```python
from build123d import *

# Parameters (mm, degrees)
SKETCH1_W           = 55
SKETCH1_H           = 25
BOSS_EXTRUDE1_DEPTH = 6
FILLET1_R           = 5


with BuildPart() as part:
    # Sketch1 → Boss-Extrude1 (new body)
    with BuildSketch(Plane.XY):
        Rectangle(SKETCH1_W, SKETCH1_H)
    extrude(amount=BOSS_EXTRUDE1_DEPTH)

    # Fillet1
    fillet1_edges = [part.edges().sort_by_distance(p)[0] for p in [
        (0, -12.5, 6),
    ]]
    fillet(fillet1_edges, radius=FILLET1_R)


solid = part.part
```
Model file for the job. Use its own axes, mm. Coordinates: 2 decimals unless noted, no trailing zeros. Write each loop counter-clockwise with the first axis right and the second up, starting at its lowest first coordinate (ties: lowest second). Pieces come first, ordered by that corner, then holes. Notation, with made-up numbers: (-11, -36) - (-2, -36) arc R17 cw to (-2, -24) - close; hole circle Ø3 at (27, 30). An arc over 180 degrees is marked (long way). One line per item, written item: value. Start each with the question number.
1. Slice it at A-A (x = -13). Write the cut outline in (y, z).
2. Flat gauge pin, fed straight in: pin 1 (1 mm diameter, centred on x = -13.5, z = 2.5, fed in from -Y). Where does the tip first touch, or does it go through?
3. Slice it at B-B (z = 5). Write the cut outline in (x, y), plus the area to 4 significant figures.
4. Probe line 1 (Y direction, x = 3.5, z = 3); line 2 (Z direction, x = 4.5, y = -11); line 3 (Y direction, x = 5, z = 3.75). List the from-to ranges inside material, lowest first. Write a range as from..to.
Answers below:
1. outline: (-12.5, 0) - (12.5, 0) - (12.5, 6) - (-7.5, 6) arc R5 ccw to (-12.5, 1) - close
2. pin 1: stops at y = -12.4
3. outline: (-27.5, -10.5) - (27.5, -10.5) - (27.5, 12.5) - (-27.5, 12.5) - close
3. area: 1,265 mm^2
4. line 1: y = -12.08..12.5
4. line 2: z = 0..4.57
4. line 3: y = -11.68..12.5
